Input: dimensioned drawing with shaded views. Units: mm. Origin: part minimum x, y, z. Give positions to 0.01 mm unless a question says otherwise; leave off trailing zeros. Loops run counter-clockwise (first coordinate to the right, second up) from the corner with the lowest first, then second, coordinate; pieces in that order, holes last.
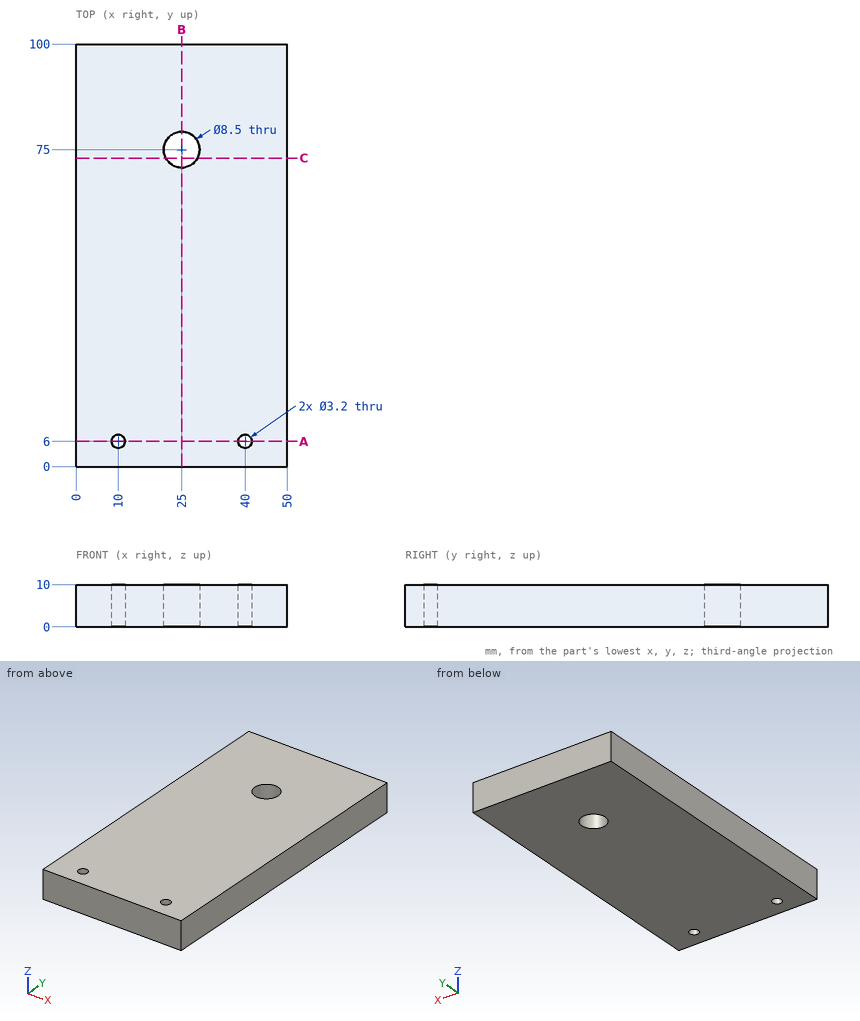
Item 1: Pin query (flat end, axial travel): pin 1 (2.5 mm diameter, centred on x = 10, y = 6, fed in from +Z). Return the tip coordinate at first contact, or that it passes through.
Values follow:
pin 1: passes through
Item 2: Section query C-C on y = 73. Return loops of the section in (x, z), plus the area to 3 significant figures.
Values follow:
outline: (0, 0) - (21.25, 0) - (21.25, 10) - (0, 10) - close; (28.75, 0) - (50, 0) - (50, 10) - (28.75, 10) - close
area: 425 mm2
Item 3: Section query B-B on x = 25. Return loops of the section in (y, z), plus the area to 3 significant figures.
Values follow:
outline: (0, 0) - (70.75, 0) - (70.75, 10) - (0, 10) - close; (79.25, 0) - (100, 0) - (100, 10) - (79.25, 10) - close
area: 915 mm2
Item 4: Ray query, probe 1 along X at (y, z) = (6, 5.75); probe 2 along Y at (x, z) = (25, 7); probe 3 along Y at (x, z) = (10, 3). Return the intervals inside material, ascending.
Values follow:
probe 1: x = 0 to 8.4, 11.6 to 38.4, 41.6 to 50
probe 2: y = 0 to 70.75, 79.25 to 100
probe 3: y = 0 to 4.4, 7.6 to 100
Item 5: Section query A-A on y = 6. Return loops of the section in (x, z), plus the area to 3 significant figures.
Values follow:
outline: (0, 0) - (8.4, 0) - (8.4, 10) - (0, 10) - close; (11.6, 0) - (38.4, 0) - (38.4, 10) - (11.6, 10) - close; (41.6, 0) - (50, 0) - (50, 10) - (41.6, 10) - close
area: 436 mm2
